```python
from build123d import *

# Parameters (mm, degrees)
BOSS_EXTRUDE1_DEPTH      = 63.5
BOSS_EXTRUDE1_DEPTH_BACK = 63.5
SKETCH3_R                = 36.5125
BOSS_EXTRUDE2_DEPTH      = 101.6
SKETCH4_R                = 19.304
CUT_EXTRUDE1_DEPTH       = 128
SKETCH5_R                = 25.654
CUT_EXTRUDE2_DEPTH       = 12.7
SKETCH6_R                = 25.654
CUT_EXTRUDE3_DEPTH       = 12.7
SKETCH7_R                = 30.4165
CUT_EXTRUDE4_DEPTH       = 78.834
CHAMFER1_SIZE            = 19.05
FILLET1_R                = 10
FILLET2_R                = 1.5875
SKETCH8_W                = 121.091569705
SKETCH8_H                = 140.894572221
CUT_EXTRUDE5_DEPTH       = 37.5125001
CUT_EXTRUDE5_DEPTH_BACK  = 37.5125


with BuildPart() as part:
    # Sketch1 → Boss-Extrude1 (new body, two sides)
    with BuildSketch(Plane.XY) as boss_extrude1_sk:
        with BuildLine():
            Line((-36.5125, 0), (-36.5125, -34.845102384))
            Line((-36.5125, -34.845102384), (36.5125, -34.845102384))
            Line((36.5125, -34.845102384), (36.5125, 0))
            ThreePointArc((36.5125, 0), (0, 36.5125), (-36.5125, 0))
        make_face()
    extrude(amount=BOSS_EXTRUDE1_DEPTH)
    extrude(boss_extrude1_sk.sketch, amount=-BOSS_EXTRUDE1_DEPTH_BACK)

    # Sketch3 → Boss-Extrude2 (add)
    with BuildSketch(Plane(origin=(0, 0, 0), x_dir=(1, 0, 0), z_dir=(0, 1, 0))):
        Circle(SKETCH3_R)
    extrude(amount=BOSS_EXTRUDE2_DEPTH)

    # Sketch4 → Cut-Extrude1 (cut, through all)
    with BuildSketch(Plane(origin=(0, 0, -63.5), x_dir=(-1, 0, 0), z_dir=(0, 0, -1))):
        Circle(SKETCH4_R)
    extrude(amount=-CUT_EXTRUDE1_DEPTH, mode=Mode.SUBTRACT)

    # Sketch5 → Cut-Extrude2 (cut)
    with BuildSketch(Plane(origin=(0, 0, -63.5), x_dir=(-1, 0, 0), z_dir=(0, 0, -1))):
        Circle(SKETCH5_R)
    extrude(amount=-CUT_EXTRUDE2_DEPTH, mode=Mode.SUBTRACT)

    # Sketch6 → Cut-Extrude3 (cut)
    with BuildSketch(Plane.XY.offset(63.5)):
        Circle(SKETCH6_R)
    extrude(amount=-CUT_EXTRUDE3_DEPTH, mode=Mode.SUBTRACT)

    # Sketch7 → Cut-Extrude4 (cut)
    with BuildSketch(Plane(origin=(0, 101.6, 0), x_dir=(1, 0, 0), z_dir=(0, 1, 0))):
        Circle(SKETCH7_R)
    extrude(amount=-CUT_EXTRUDE4_DEPTH, mode=Mode.SUBTRACT)

    # Chamfer1
    chamfer1_edges = [part.edges().sort_by_distance(p)[0] for p in [
        (-36.5125, -34.845102384, 0),
        (36.5125, -34.845102384, 0),
    ]]
    chamfer(chamfer1_edges, length=CHAMFER1_SIZE)

    # Fillet1
    fillet1_edges = [part.edges().sort_by_distance(p)[0] for p in [
        (-17.4625, -34.845102384, 0),
        (17.4625, -34.845102384, 0),
        (36.5125, -15.795102384, 0),
        (-36.5125, -15.795102384, 0),
    ]]
    fillet(fillet1_edges, radius=FILLET1_R)

    # Fillet2
    fillet2_edges = [part.edges().sort_by_distance(p)[0] for p in [
        (-36.5125, -5.82648338, -63.5),
        (36.5125, -5.82648338, 63.5),
        (0, 36.5125, 63.5),
        (-36.5125, -5.82648338, 63.5),
        (0, 36.5125, -63.5),
        (-36.5125, 101.6, 0),
        (19.304, 0, -50.8),
        (36.5125, -5.82648338, -63.5),
        (19.304, 0, 50.8),
        (-30.4165, 101.6, 0),
        (26.9875, -25.320102384, -63.5),
        (0, -34.845102384, -63.5),
        (-26.9875, -25.320102384, -63.5),
        (-35.751295325, -15.479801084, -63.5),
        (-17.1471987, -34.083897709, -63.5),
        (17.1471987, -34.083897709, -63.5),
        (35.751295325, -15.479801084, -63.5),
        (26.9875, -25.320102384, 63.5),
        (0, -34.845102384, 63.5),
        (-26.9875, -25.320102384, 63.5),
        (-35.751295325, -15.479801084, 63.5),
        (-17.1471987, -34.083897709, 63.5),
        (17.1471987, -34.083897709, 63.5),
        (35.751295325, -15.479801084, 63.5),
    ]]
    fillet(fillet2_edges, radius=FILLET2_R)

    # Sketch8 → Cut-Extrude5 (cut, two sides)
    with BuildSketch(Plane(origin=(0, 0, 0), x_dir=(0, 0, -1), z_dir=(1, 0, 0))) as cut_extrude5_sk:
        with Locations((-17.762374118, 35.602183727)):
            Rectangle(SKETCH8_W, SKETCH8_H)
    extrude(amount=CUT_EXTRUDE5_DEPTH, mode=Mode.SUBTRACT)
    extrude(cut_extrude5_sk.sketch, amount=-CUT_EXTRUDE5_DEPTH_BACK, mode=Mode.SUBTRACT)


solid = part.part
```
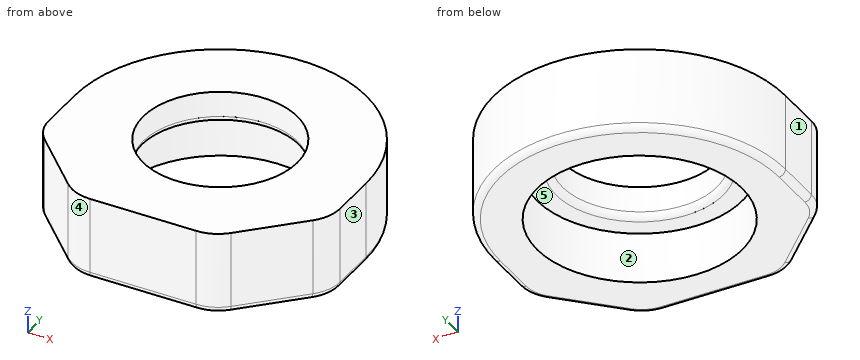
Build history of the part. All positions in model axes, mm. Face numbers are marked on the shaded views. A direction names the side the tool comes from. Coordinates: 2 decimals unless noted, no trailing zeros. Order: outer loops, then holes, each group sorted by start corner. A loop starts at its lowest first (then second) coordinate and runs counter-clockwise, first axis right, second up. Notation, with made-up numbers: M -27,20 L -11,20 A20 ccw -11,56 Z; hole C 9,-2 d6. An arc over 180 degrees is marked long. One line per question, with ' | ' between items. Start each with the question number.
1. Cut at A-A (z = -55.25). Write the cut outline in (x, y) (1 decimal).
2. Mould opens along Y. For the marked faces 3, 4 and 5 say: +Y half, -Y half, draft (parallel to the pull), parting line (faces both ways), or undercut.
3. Flat gauge pins, fed straight in: P1, Ø3, axis at x = -19, y = 12, coming from the -Z side; P2, Ø6, axis at x = -21.5, z = -57.5, coming from the -Y side; P3, Ø12, axis at x = 22, z = -48.5, coming from the -Y side; P4, Ø15.5, axis at x = -1, y = 4.5, coming from the -Z side. Where does each tip first touch, or does it go through?
4. Tool access for the marked faces 1 and 2: list every direction of +Z, -Z, +X, -X, +Y, -Y with a clear straight run to the whole face (end or side of a thin tool).
5. Wall check: line 1 along Y through (x, z) = (0, -57.75); line 2 along X through (y, z) = (-3.5, -46.5); line 3 along Z through (x, y) = (-22, -2). Give the ranges that are in metal, low to high. Write a range as [from, to].
6. Cut at B-B (x = 0). Write the cut outline in (y, z) (1 decimal).
The answers:
1) outline: M -36.5,-11.7 A10 ccw -33.6,-18.7 L -20.4,-31.9 A10 ccw -13.3,-34.8 L 13.3,-34.8 A10 ccw 20.4,-31.9 L 33.6,-18.7 A10 ccw 36.5,-11.7 L 36.5,0 A36.5 ccw -36.5,0 Z; hole C 0,0 d51.3
2) face 3: draft | face 4: -Y half | face 5: undercut
3) P1: stops at z = -50.8 | P2: stops at y = -33.4 | P3: stops at y = -34.48 | P4: passes through
4) face 1: +Z, -Z, -X, +Y, -Y | face 2: -Z
5) line 1: y = [-34.85, -25.65], [25.65, 36.51] | line 2: x = [-36.51, -18.98], [18.98, 36.51] | line 3: z = [-50.8, -42.78]
6) outline: M -34.8,-61.9 A1.6 ccw -33.3,-63.5 L -25.7,-63.5 L -25.7,-50.8 L -20.9,-50.8 A1.6 ccw -19.3,-49.2 L -19.3,-42.8 L -34.8,-42.8 Z; M 19.3,-49.2 A1.6 ccw 20.9,-50.8 L 25.7,-50.8 L 25.7,-63.5 L 34.9,-63.5 A1.6 ccw 36.5,-61.9 L 36.5,-42.8 L 19.3,-42.8 Z
